Here's the drawing with two shaded views (mm, measured from the low corner). I have some questions. Round coordinates to 2 decimals unless told otherwise and drop trailing zeros. Order: outer loops, then holes, each group sorted by start corner. A loop starts at its lowest first (then second) coordinate and runs counter-clockwise, first axis right, second up.
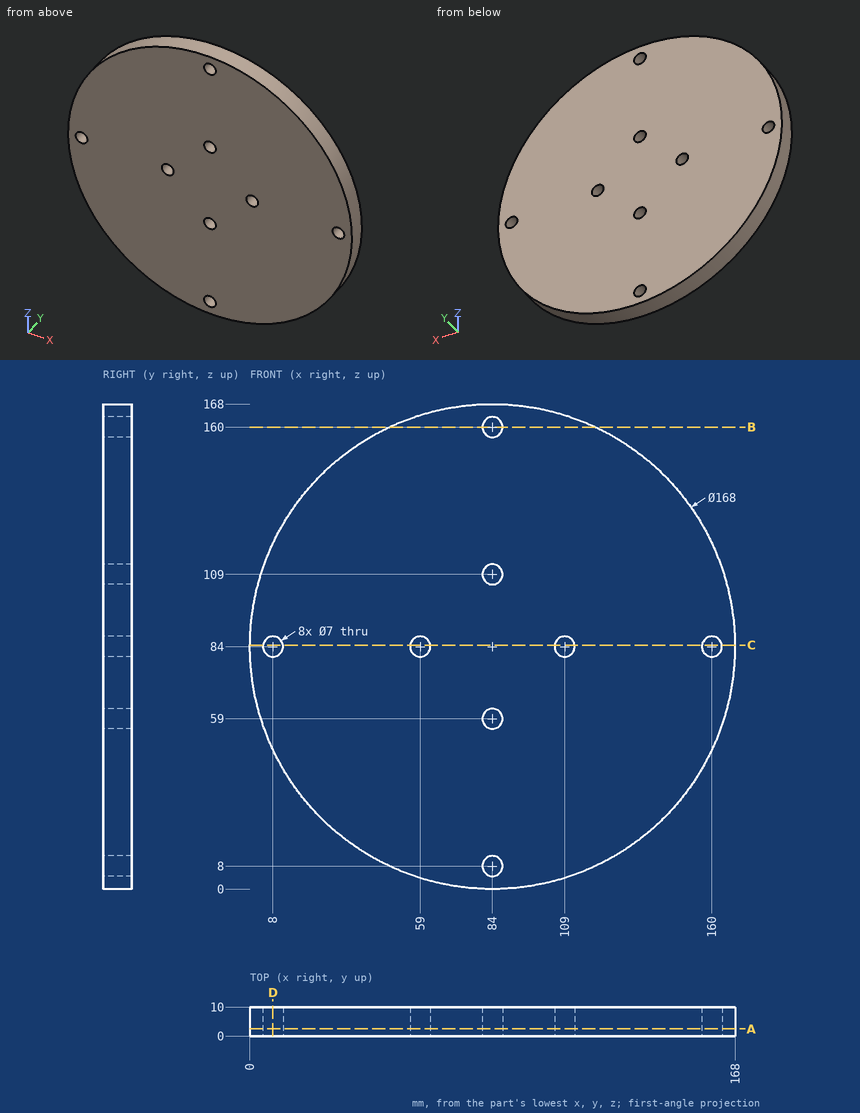
1. I'm going to push flat-ended pins straight in: P1, Ø11, axis at x = 59, z = 84, coming from the -Y side; P2, Ø5, axis at x = 66.5, y = 1, coming from the -Z side; P3, Ø4, axis at x = 84, z = 59, coming from the +Y side; P4, Ø5, axis at x = 122, y = 4, coming from the +Z side. Where does each tip first touch, or does it pass through?
Evaluation:
P1: stops at y = 0
P2: stops at z = 1.35
P3: passes through
P4: stops at z = 160.13
2. I need wall thicknesses on probe 1 along X at (y, z) = (7.25, 84); probe 2 along Z at (x, y) = (160, 3.5); probe 3 along X at (y, z) = (4.75, 109). Which ranges of each line are inside material? Lowest first, please.
Evaluation:
probe 1: x = 0 to 4.5, 11.5 to 55.5, 62.5 to 105.5, 112.5 to 156.5, 163.5 to 168
probe 2: z = 48.22 to 80.5, 87.5 to 119.78
probe 3: x = 3.81 to 80.5, 87.5 to 164.19
3. If we section it at B-B, the plane z = 160: Write out the boundary of the cut face in (x, y).
Evaluation:
outline: (48.22, 0) - (80.5, 0) - (80.5, 10) - (48.22, 10) - close; (87.5, 0) - (119.78, 0) - (119.78, 10) - (87.5, 10) - close
4. If we section it at C-C, the plane z = 84.5: Write out the boundary of the cut face in (x, y), and give its area (3 significant figures).
Evaluation:
outline: (0, 0) - (4.54, 0) - (4.54, 10) - (0, 10) - close; (11.46, 0) - (55.54, 0) - (55.54, 10) - (11.46, 10) - close; (62.46, 0) - (105.54, 0) - (105.54, 10) - (62.46, 10) - close; (112.46, 0) - (156.54, 0) - (156.54, 10) - (112.46, 10) - close; (163.46, 0) - (168, 0) - (168, 10) - (163.46, 10) - close
area: 1,400 mm2
5. If we section it at A-A, the plane y = 2.5: State how many separate pieces and enclosed holes the cut face has, and give its area (3 significant figures).
Evaluation:
separate pieces: 1
enclosed holes: 8
area: 21,900 mm2
6. If we section it at D-D, the plane x = 8: Write out the boundary of the cut face in (y, z), and give its area (3 significant figures).
Evaluation:
outline: (0, 48.22) - (10, 48.22) - (10, 80.5) - (0, 80.5) - close; (0, 87.5) - (10, 87.5) - (10, 119.78) - (0, 119.78) - close
area: 646 mm2
